Could you check a few things on this model? Use its own coordinates, in mm. A direction names the side the tool comes from. Give positions to 0.01 mm unless a question says otherwise; leave off trailing zeros. Order: outer loops, then holes, each group sorted by start corner. A loop starts at its lowest first (then second) coordinate and runs counter-clockwise, first axis right, second up. Notation, with made-up numbers: M 70.25,28 L 96.25,28 A10 ccw 96.25,32 Z; hole C 5.25,47.5 d11. An arc over 180 degrees is marked long. Use a Markdown table: item, result. Add a question column.
```python
from build123d import *

# Parameters (mm, degrees)
F0_R     = 11.05
F1_DEPTH = 2.1
F2_R     = 4.5
F3_DEPTH = 1.11
F6_DEPTH = 6
F7_W     = 2.7
F7_H     = 1.5
F8_DEPTH = 1
F9_SIZE  = 0.3
F10_SIZE = 0.5


# Not quite as in the source:
# - two fillets or chamfers of one size are made in one step


with BuildPart() as f1:
    # F0 (on Top) → F1 (new body)
    with BuildSketch(Plane.XY):
        Circle(F0_R)
    extrude(amount=F1_DEPTH)

    # F2 (on face) → F3 (join)
    with BuildSketch(Plane.XY.offset(2.1)):
        Circle(F2_R)
    extrude(amount=F3_DEPTH)

    # F5 (on face) → F6 (join)
    with BuildSketch(Plane.XY.offset(3.21)):
        Polygon((-1.35, -2), (1.35, -2), (1.35, 0), (1.35, 1), (-1.35, 1), (-1.35, 0), align=None)
    extrude(amount=F6_DEPTH)

    # F7 (on face) → F8 (join)
    with BuildSketch(Plane(origin=(0, 1, 0), x_dir=(-1, 0, 0), z_dir=(0, 1, 0))):
        with Locations((0, 8.46)):
            Rectangle(F7_W, F7_H)
    extrude(amount=F8_DEPTH)

    # F9
    f9_edges = [f1.edges().sort_by_distance(p)[0] for p in [
        (-1.35, -2, 6.21),
        (1.35, -2, 6.21),
        (1.35, 1, 5.46),
        (-1.35, 1, 5.46),
        (1.35, 1.5, 7.71),
        (-1.35, 1.5, 7.71),
        (0, 2, 7.71),
        (1.35, 2, 8.46),
        (-1.35, 2, 8.46),
        (0, 2, 9.21),
        (1.35, 0, 9.21),
        (-1.35, 0, 9.21),
        (0, -2, 9.21),
        (-1.35, -0.5, 3.21),
        (0, -2, 3.21),
        (1.35, -0.5, 3.21),
        (0, 1, 3.21),
    ]]
    chamfer(f9_edges, length=F9_SIZE)

    # F10
    f10_edges = [f1.edges().sort_by_distance(p)[0] for p in [
        (-11.05, 0, 0),
        (-11.05, 0, 2.1),
    ]]
    chamfer(f10_edges, length=F10_SIZE)


solid = f1.part
```
1) For faces 1 (the face through (5, 0, 2.1)), 2 (the face through (-1.35, 0, 6)), 3 (the face through (0, -2, 6)), which set-ups out of +Z, -Z, +X, -X, +Y, -Y let a thin tool reach every point of the face, with its end or its side?
2) Suppose I cut it at B-B on x = 0. Please give me the cut outline in (y, z).
3) Suppose I cut it at A-A on y = 0. Please give me the cut outline in (x, z).
4) Please list where these lines run through material, in increasing order: line 1 (Z direction, x = 3.75, y = 4.25); line 2 (Z direction, x = 3.75, y = 0); line 3 (Y direction, x = -0.25, z = 4.25). Write a range as from..to.
5) We'd pull the mould along Z, two halves only. Please class faces 4 (the face through (0, 0, 9.21)), 5 (the face through (0, 2, 8.5)), 6 (the face through (0, 1, 6)), 7 (the face through (0, 0, 0)): pulls with the +Z half, pulls with the -Z half, needs draft (parallel to the pull), parting line crosses it, or undercut.
6) Suppose I cut it at D-D on z = 2.75. Please give me the cut outline in (x, y), and give its area (3 significant figures).
7) For pin 1 (1 mm diameter, centred on y = -8.5, z = 1, fed in from -X); pin 2 (2.5 mm diameter, centred on x = 0.5, z = 5, fed in from +Y); pin 3 (3 mm diameter, centred on x = -0.5, z = 7, fed in from +Y), each with a flat end and sliding along its axis, tell me the tip position at first contact or that it passes through.
8) Suppose I cut it at C-C on z = 1.25. Please give me the cut outline in (x, y).
Values found:
| question | item | result |
|---|---|---|
| 1 | face 1 | +Z |
| 1 | face 2 | +Z, -X, +Y, -Y |
| 1 | face 3 | +Z, +X, -X, -Y |
| 2 | outline | M -11.05,0.5 L -10.55,0 L 10.55,0 L 11.05,0.5 L 11.05,1.6 L 10.55,2.1 L 4.5,2.1 L 4.5,3.21 L 1.3,3.21 L 1,3.51 L 1,7.71 L 1.7,7.71 L 2,8.01 L 2,8.91 L 1.7,9.21 L -1.7,9.21 L -2,8.91 L -2,3.51 L -2.3,3.21 L -4.5,3.21 L -4.5,2.1 L -10.55,2.1 L -11.05,1.6 Z |
| 3 | outline | M -11.05,0.5 L -10.55,0 L 10.55,0 L 11.05,0.5 L 11.05,1.6 L 10.55,2.1 L 4.5,2.1 L 4.5,3.21 L 1.65,3.21 L 1.35,3.51 L 1.35,8.91 L 1.05,9.21 L -1.05,9.21 L -1.35,8.91 L -1.35,3.51 L -1.65,3.21 L -4.5,3.21 L -4.5,2.1 L -10.55,2.1 L -11.05,1.6 Z |
| 4 | line 1 | z = 0..2.1 |
| 4 | line 2 | z = 0..3.21 |
| 4 | line 3 | y = -2..1 |
| 5 | face 4 | pulls with the +Z half |
| 5 | face 5 | needs draft |
| 5 | face 6 | undercut |
| 5 | face 7 | pulls with the -Z half |
| 6 | outline | C 0,0 d9 |
| 6 | area | 63.6 mm^2 |
| 7 | pin 1 | stops at x = -7.62 |
| 7 | pin 2 | stops at y = 1 |
| 7 | pin 3 | stops at y = 2 |
| 8 | outline | C 0,0 d22.1 |
